Part print with two shaded views. Sizes in mm from the minimum x, y, z corner. A direction names the side the tool comes from. Coordinates: 2 decimals unless noted, no trailing zeros. Loops run counter-clockwise (first coordinate to the right, second up) from the corner with the lowest first, then second, coordinate; pieces in that order, holes last.
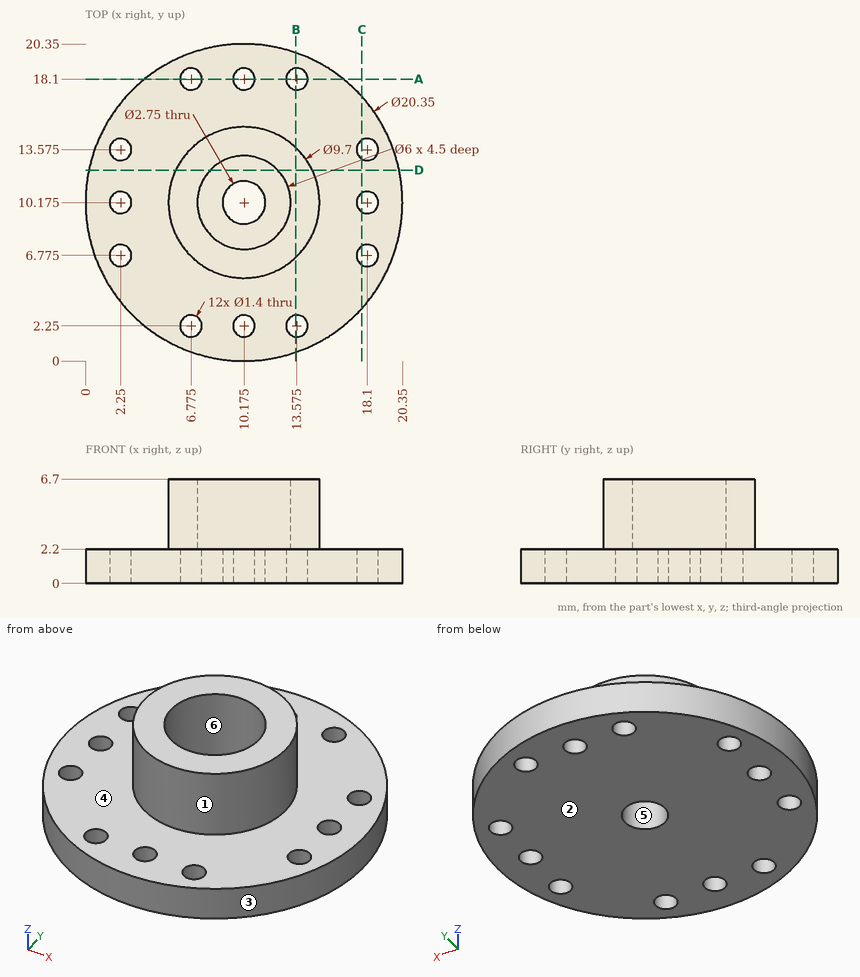
Q1. Flat gauge pins, fed straight in: P1, Ø2, axis at x = 10.175, y = 18.1, coming from the +Z side; P2, Ø2, axis at x = 13, z = 2.5, coming from the +Y side; P3, Ø4, axis at x = 3, z = 1, coming from the +Y side. Where does each tip first touch, or does it go through?
Answers:
P1: stops at z = 2.2
P2: stops at y = 20.18
P3: stops at y = 18.94
Q2. Slice it at B-B (x = 13.5). List the corners of the cut face in (y, z), and give its area (3 significant figures).
Answers:
outline: (0.56, 0) - (1.55, 0) - (1.55, 2.2) - (0.56, 2.2) - close; (2.95, 0) - (17.4, 0) - (17.4, 2.2) - (13.71, 2.2) - (13.71, 6.7) - (6.64, 6.7) - (6.64, 2.2) - (2.95, 2.2) - close; (18.8, 0) - (19.79, 0) - (19.79, 2.2) - (18.8, 2.2) - close
area: 68.0 mm2
Q3. Mould opens along X. For the marked faces 3, 4, 5 and 6 say: +X half, -X half, draft (parallel to the pull), parting line (faces both ways), or undercut.
Answers:
face 3: parting line
face 4: draft
face 5: undercut
face 6: undercut
Q4. Slice it at A-A (y = 18.1). List the corners of the cut face in (x, z) (3 decimals), and give its area (3 significant figures).
Answers:
outline: (3.793, 0) - (6.075, 0) - (6.075, 2.2) - (3.793, 2.2) - close; (7.475, 0) - (9.475, 0) - (9.475, 2.2) - (7.475, 2.2) - close; (10.875, 0) - (12.875, 0) - (12.875, 2.2) - (10.875, 2.2) - close; (14.275, 0) - (16.557, 0) - (16.557, 2.2) - (14.275, 2.2) - close
area: 18.8 mm2
Q5. Which spindle directions (+Z, -Z, +X, -X, +Y, -Y) get a long thin tool onto all of the face, cutting with end or side? Do the marked faces 1 and 2. Say none if no direction does.
Answers:
face 1: +Z
face 2: -Z, +X, -X, +Y, -Y
Q6. Slice it at D-D (y = 12.25). List the corners of the cut face in (x, z), and give its area (3 significant figures).
Answers:
outline: (0.21, 0) - (20.14, 0) - (20.14, 2.2) - (14.56, 2.2) - (14.56, 6.7) - (12.34, 6.7) - (12.34, 2.2) - (8.01, 2.2) - (8.01, 6.7) - (5.79, 6.7) - (5.79, 2.2) - (0.21, 2.2) - close
area: 63.8 mm2
Q7. Drill centre lines: line 1 (Y direction, x = 18.1, z = 1.45) (3 decimals); line 2 (X direction, y = 18, z = 0.75). Where is each one in solid material? Low to high.
Answers:
line 1: y = 3.793 to 6.075, 7.475 to 9.475, 10.875 to 12.875, 14.275 to 16.557
line 2: x = 3.67 to 6.08, 7.47 to 9.48, 10.87 to 12.88, 14.27 to 16.68
Q8. Slice it at C-C (x = 17.75). List the corners of the cut face in (y, z).
Answers:
outline: (3.38, 0) - (6.17, 0) - (6.17, 2.2) - (3.38, 2.2) - close; (7.38, 0) - (9.57, 0) - (9.57, 2.2) - (7.38, 2.2) - close; (10.78, 0) - (12.97, 0) - (12.97, 2.2) - (10.78, 2.2) - close; (14.18, 0) - (16.97, 0) - (16.97, 2.2) - (14.18, 2.2) - close
